Source: three-view drawing plus pictorial views. Frame: mm from the lowest corner of the part. A direction names the side the tool comes from. Round coordinates to 2 decimals unless told otherwise and drop trailing zeros. Order: outer loops, then holes, each group sorted by start corner. A loop starts at its lowest first (then second) coordinate and runs counter-clockwise, first axis right, second up. Notation, with made-up numbers: M -26,55 L 15,55 A29 cw 15,78 Z; hole C 47.5,33.25 d7. An arc over 180 degrees is marked long. Return JSON: item names as keys, results as strings. Group by question number.
Q1. Ray query, probe 1 along X at (y, z) = (2.25, 20); probe 2 along Y at (x, z) = (47.65, 60); probe 3 along Z at (x, y) = (37, 4.3). Return the intervals inside material, ascending.
Q2. Cut plane A-A on z = 60. Output: boundary loops of the cut face in (x, y), and give its area (3 significant figures).
Q3. Cut plane C-C on y = 57. Output: boundary loops of the cut face in (x, z), and give its area (3 significant figures).
Q4. Cut plane D-D on z = 14. Output: boundary loops of the cut face in (x, y).
Q5. Contact query for flat-ended pins moving along their axis: pin 1 (3.5 mm diameter, centred on x = 47, y = 17, fed in from +Z); pin 2 (6.5 mm diameter, centred on x = 37, z = 100, fed in from +Y); pin 3 (1 mm diameter, centred on y = 66, z = 81, fed in from -X). Output: stop coordinate, or through.
Q6. Cut plane B-B on y = 49.5. Output: boundary loops of the cut face in (x, z), and give its area (3 significant figures).
Q7. Access query for the marked faces 1 and 2. Directions: +Z, -Z, +X, -X, +Y, -Y. A direction counts if a zero-diameter tool reaches every point of the face in a straight line with its end or side. Return the directions, or none.
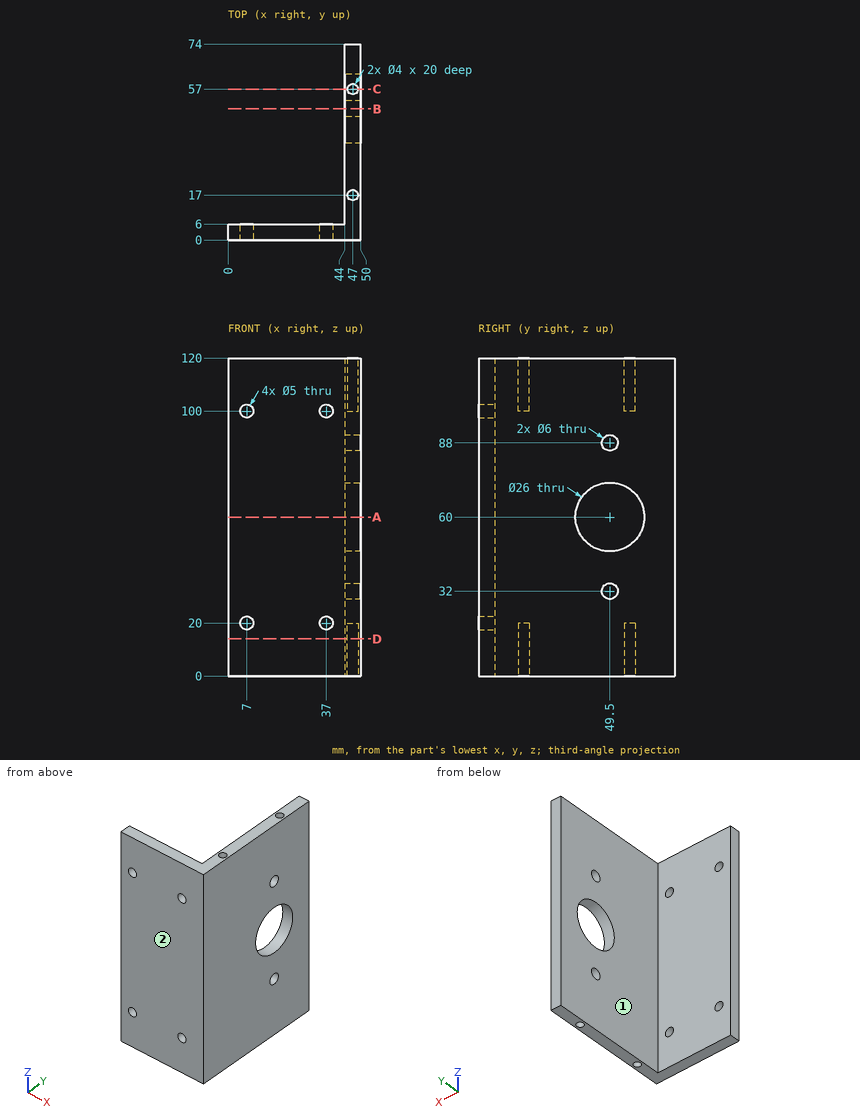
Result sheet:
{
 "1": {"probe 1": "x = 0 to 4.5, 9.5 to 34.5, 39.5 to 50", "probe 2": "y = 0 to 36.5, 62.5 to 74", "probe 3": "z = 0 to 17.5, 22.5 to 97.5, 102.5 to 120"},
 "2": {"outline": "M 0,0 L 50,0 L 50,36.5 L 44,36.5 L 44,6 L 0,6 Z; M 44,62.5 L 50,62.5 L 50,74 L 44,74 Z", "area": "552 mm²"},
 "3": {"outline": "M 44,0 L 45,0 L 45,20 L 49,20 L 49,0 L 50,0 L 50,49.38 L 44,49.38 Z; M 44,70.62 L 50,70.62 L 50,120 L 49,120 L 49,100 L 45,100 L 45,120 L 44,120 Z", "area": "433 mm²"},
 "4": {"outline": "M 0,0 L 50,0 L 50,74 L 44,74 L 44,6 L 0,6 Z; hole C 47,17 d4; hole C 47,57 d4"},
 "5": {"pin 1": "stops at z = 100", "pin 2": "stops at y = 6", "pin 3": "stops at x = 44"},
 "6": {"outline": "M 44,0 L 50,0 L 50,29 L 44,29 Z; M 44,35 L 50,35 L 50,47 L 44,47 Z; M 44,73 L 50,73 L 50,85 L 44,85 Z; M 44,91 L 50,91 L 50,120 L 44,120 Z", "area": "492 mm²"},
 "7": {"face 1": "+Z, -Z, -X, +Y", "face 2": "+Z, -Z, +X, -X, -Y"}
}
